Can you work these out from the drawing? Everything is in mm from the part's minimum corner. A direction names the side the tool comes from. Coordinates: 2 decimals unless noted, no trailing zeros. Order: outer loops, then holes, each group sorted by start corner. A loop starts at its lowest first (then second) coordinate and runs counter-clockwise, first axis right, second up. Notation, with made-up numbers: (-22, 75.5) - (6, 75.5) arc R28 cw to (6, 111.5) - close; hole circle Ø3 at (8.5, 86). An arc over 180 degrees is marked (long way). Use a Markdown table: item, result. Add a question column.
(1) I want a section at A-A (y = 16). List the corners of the cut face in (x, z) for me, and give its area (3 significant figures).
(2) I want a section at C-C (x = 10.25). List the corners of the cut face in (y, z) for me.
(3) On a 3-axis mill with a long thin cutter (end or side, diameter ignored), from which of +Z, -Z, +X, -X, +Y, -Y can I reach the whole of each face in a straight line? I mean the marked faces 4 and 5. Say none if no direction works.
(4) I want a section at B-B (z = 24). List the corners of the cut face in (x, y) for me, and give its area (3 significant figures).
(5) If I drill on L1, parallel to X at y = 8, z = 15; L2, parallel to Z at x = 3, y = 15.75; L3, parallel to Y at x = 3.25, z = 11.5, over which ranges is the centre line in solid material (lowest first)? Write a range as [from, to].
(6) For pin 1 Ø6.5 at (x, y) = (6, 6.5) entering from -Z; pin 2 Ø5 at (x, z) = (10, 19.5) entering from +Y, each with a flat end and sliding along its axis, tell me the tip position at first contact or that it passes through.
(7) We'd pull the mould along X, two halves only. Please class the marked faces 1, 2 and 3: pulls with the +X half, pulls with the -X half, needs draft (parallel to the pull), parting line crosses it, or undercut.
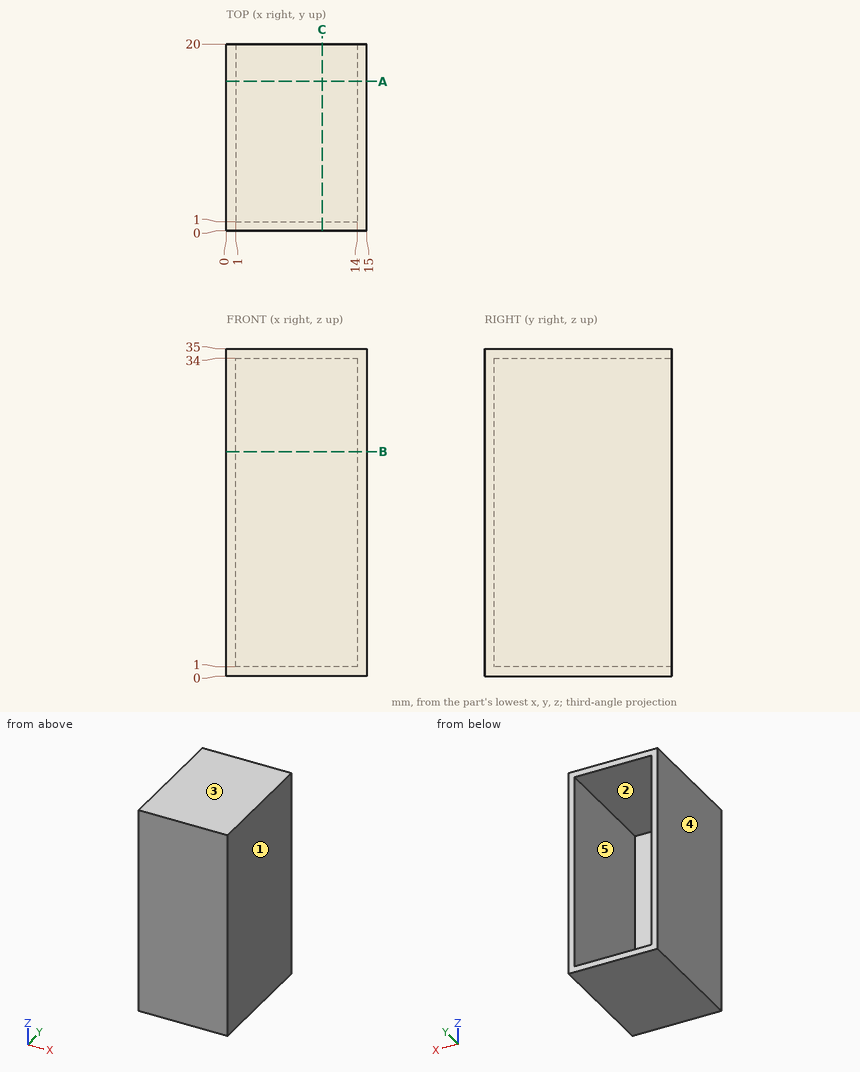
Answers follow:
| question | item | result |
|---|---|---|
| 1 | outline | (0, 0) - (15, 0) - (15, 35) - (0, 35) - close; hole (1, 1) - (14, 1) - (14, 34) - (1, 34) - close |
| 1 | area | 96.0 mm² |
| 2 | outline | (0, 0) - (20, 0) - (20, 1) - (1, 1) - (1, 34) - (20, 34) - (20, 35) - (0, 35) - close |
| 3 | face 4 | +Z, -Z, -X, +Y, -Y |
| 3 | face 5 | +Y |
| 4 | outline | (0, 0) - (15, 0) - (15, 20) - (14, 20) - (14, 1) - (1, 1) - (1, 20) - (0, 20) - close |
| 4 | area | 53.0 mm² |
| 5 | L1 | x = [0, 1], [14, 15] |
| 5 | L2 | z = [0, 1], [34, 35] |
| 5 | L3 | y = [0, 1] |
| 6 | pin 1 | stops at z = 0 |
| 6 | pin 2 | stops at y = 1 |
| 7 | face 1 | pulls with the +X half |
| 7 | face 2 | undercut |
| 7 | face 3 | needs draft |
